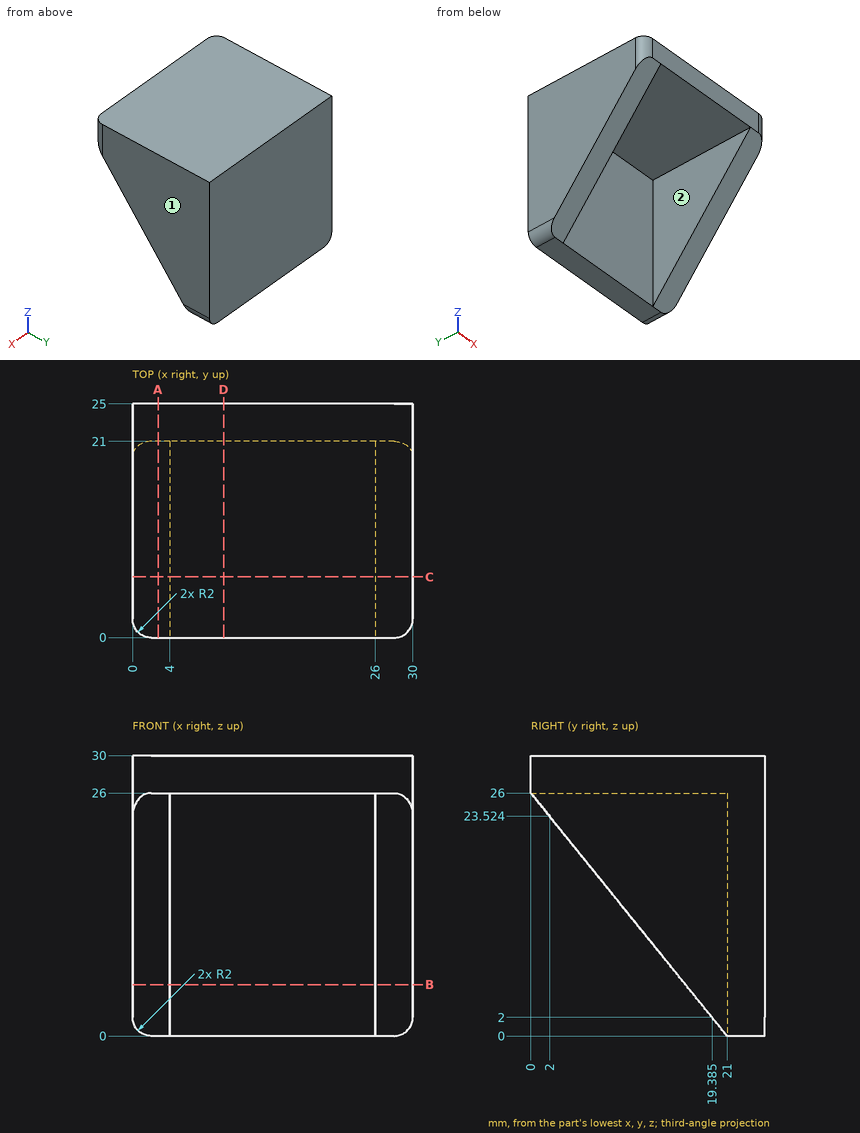
Could you check a few things on this drawing? It's one solid part, dimensions in mm from its lowest x, y, z. A direction names the side the tool comes from. Coordinates: 2 decimals unless noted, no trailing zeros. Order: outer loops, then holes, each group sorted by start corner. A loop starts at its lowest first (then second) coordinate and runs counter-clockwise, first axis right, second up. Notation, with made-up numbers: (-33.5, 28) - (-11.5, 28) arc R10 ccw to (-11.5, 39) - close; hole circle Ø3 at (-5, 79.25). An arc over 180 degrees is marked (long way). Answer as a JSON object with one key per item and string values. Group by question number.
Q1. On a 3-axis mill with a long thin cutter (end or side, diameter ignored), from which of +Z, -Z, +X, -X, +Y, -Y can I reach the whole of each face in a straight line? I mean the marked faces 1 and 2. Say none if no direction works.
Q2. Imagine slicing it at A-A (x = 2.75). Please give me the cut outline in (y, z), and give its area (3 significant figures).
Q3. I need wall thicknesses on line 1 (X direction, y = 11, z = 21.5); line 2 (Z direction, x = 6.25, y = 13); line 3 (Y direction, x = 5.75, z = 11). Which ranges of each line are inside material? Lowest first, please. Write a range as from..to.
Q4. Imagine slicing it at B-B (z = 5.5). Please give me the cut outline in (x, y).
Q5. Imagine slicing it at C-C (y = 6.5). Please give me the cut outline in (x, z), and give its area (3 significant figures).
Q6. Will these pins go through, and if not, where does the flat tip stop? P1, Ø1, axis at x = 8.5, y = 7.5, coming from the -Z side; P2, Ø10.5, axis at y = 11, z = 10, coming from the +X side; P3, Ø3, axis at x = 8, z = 15.5, coming from the -Y side.
Q7. Imagine slicing it at D-D (x = 9.75). Please give me the cut outline in (y, z).
Determined:
{
 "1": {"face 1": "+Z, -Z, +X, +Y, -Y", "face 2": "-Z, -Y"},
 "2": {"outline": "(0, 26) - (21, 0) - (25, 0) - (25, 30) - (0, 30) - close", "area": "477 mm2"},
 "3": {"line 1": "x = 0..4, 26..30", "line 2": "z = 26..30", "line 3": "y = 21..25"},
 "4": {"outline": "(0, 16.56) - (4, 16.56) - (4, 21) - (26, 21) - (26, 16.56) - (30, 16.56) - (30, 25) - (0, 25) - close"},
 "5": {"outline": "(0, 17.95) - (4, 17.95) - (4, 26) - (26, 26) - (26, 17.95) - (30, 17.95) - (30, 30) - (0, 30) - close", "area": "184 mm2"},
 "6": {"P1": "stops at z = 26", "P2": "stops at x = 30", "P3": "stops at y = 21"},
 "7": {"outline": "(0, 26) - (21, 26) - (21, 0) - (25, 0) - (25, 30) - (0, 30) - close"}
}
